Check sheet for the modelled part. Datum: model origin and axes. Units: mm. A direction names the side the tool comes from. Round coordinates to 2 decimals unless told otherwise and drop trailing zeros. Loops run counter-clockwise (first coordinate to the right, second up) from the corner with the lowest first, then second, coordinate; pieces in that order, holes last. Notation, with made-up numbers: (33.5, 43) - (92.5, 43) arc R24 ccw to (92.5, 69) - close; hole circle Ø8 at (24.5, -33.5). An arc over 180 degrees is marked (long way). Answer in a Markdown table with one row per item. Add a question column.
(1) Cross-section at C-C on y = 53. Enter the section's corners in (x, z) (3 decimals), then the cut area to 3 significant figures.
(2) Cross-section at A-A on z = 5. Enter the section's corners in (x, y) (3 decimals), then the cut area to 3 significant figures.
(3) Mould release check, pull along X, two halves, no side actions. Record for faces 5 (the flat face through (0, -63.5, 0)), 6 (the flat face through (-41.275, -1, 0)), 7 (the cylindrical face through (42.6, -0.4, 41.4)): +X half, -X half, draft (parallel to the pull), parting line (faces both ways), or undercut.
(4) Gauge pin test, flat ends, axial feed: pin 1 (4 mm diameter, centred on y = -5.5, z = 41.5, fed in from +X); pin 2 (2.5 mm diameter, centred on x = 85, y = -0.5, fed in from -Z); pin 3 (1.5 mm diameter, centred on y = 18.5, z = 41, fed in from -X). Record the tip position at first contact, or that the pin passes through.
(5) Access from +Z, -Z, +X, -X, +Y, -Y to the whole of each face (thin tool, end or side, straight path). Record for faces 1 (the flat face through (57, 0, 42.875)), 2 (the flat face through (80, 0, 38.1)), 3 (the flat face through (47, 25.4, 48)), 4 (the cylindrical face through (29.39, -16.79, 55.13)).
(6) Thickness scan on line 1 along Z through (x, y) = (34.5, -50) (3 decimals); line 2 along Y through (x, z) = (25, 45); line 3 along X through (y, z) = (9, 27.5) (3 decimals). Record the ranges inside material, lowest first.
(7) Cross-section at D-D on y = -10. Enter the section's corners in (x, z) (3 decimals), then the cut area to 3 significant figures.
(8) Cross-section at B-B on x = 65. Enter the section's corners in (y, z) (1 decimal), then the cut area to 3 significant figures.
from build123d import *

# Parameters (mm, degrees)
F1_DEPTH = 63.5
F2_DEPTH = 25.4
F3_DEPTH = 7.9375
F5_R     = 6.35


with BuildPart() as f1:
    # F0 (on Front) → F1 (new body, symmetric)
    with BuildSketch(Plane.XZ):
        Polygon((41.275, -9.525), (41.275, 9.525), (22.225, 9.525), (-41.275, 9.525), (-41.275, -9.525), align=None)
    extrude(amount=F1_DEPTH, both=True)

    # F0 (on Front) → F2 (join, symmetric)
    with BuildSketch(Plane.XZ):
        with BuildLine():
            Line((22.225, 9.525), (41.275, 9.525))
            Line((41.275, 9.525), (41.275, 38.1))
            ThreePointArc((41.275, 38.1), (42.673624, 41.476576), (46.0502, 42.8752))
            Line((46.0502, 42.8752), (60.325, 42.8752))
            Line((60.325, 42.8752), (60.325, 61.9252))
            Line((60.325, 61.9252), (46.0502, 61.9252))
            ThreePointArc((46.0502, 61.9252), (29.20324, 54.94696), (22.225, 38.1))
            Line((22.225, 38.1), (22.225, 9.525))
        make_face()
        Polygon((60.325, 61.9252), (60.325, 42.8752), (76.285926, 42.8752), (86.96812, 42.8752), (85.725, 61.9252), align=None)
    extrude(amount=F2_DEPTH, both=True)

    # F0 (on Front) → F3 (join, symmetric)
    with BuildSketch(Plane.XZ):
        with BuildLine():
            Line((-41.275, 9.525), (22.225, 9.525))
            Line((22.225, 9.525), (22.225, 38.1))
            ThreePointArc((22.225, 38.1), (29.20324, 54.94696), (46.0502, 61.9252))
            add(Edge.make_bspline(
                [(-41.275, 9.525), (-12.033702, 9.525), (10.122908, 69.295764), (46.0502, 61.9252)],
                knots=[0, 0, 0, 0, 101.840422, 101.840422, 101.840422, 101.840422], degree=3))
        make_face()
    extrude(amount=F3_DEPTH, both=True)

    # F0 (on Front) → F4 (revolve)
    with BuildSketch(Plane.XZ):
        Polygon((85.725, 66.675), (85.725, 61.9252), (86.96812, 42.8752), (86.96812, 38.1), (111.125, 38.1), (111.125, 66.675), align=None)
    revolve(axis=Axis((85.725, 0, 64.3001), (0, 0, 1)))

    # F5
    f5_edges = [f1.edges().sort_by_distance(p)[0] for p in [
        (-41.275, -63.5, 0),
        (41.275, -63.5, 0),
        (41.275, 63.5, 0),
        (-41.275, 63.5, 0),
    ]]
    fillet(f5_edges, radius=F5_R)


solid = f1.part
Answers:
| question | item | result |
|---|---|---|
| 1 | outline | (-41.275, -9.525) - (41.275, -9.525) - (41.275, 9.525) - (-41.275, 9.525) - close |
| 1 | area | 1,570 mm^2 |
| 2 | outline | (-41.275, -57.15) arc R6.35 ccw to (-34.925, -63.5) - (34.925, -63.5) arc R6.35 ccw to (41.275, -57.15) - (41.275, 57.15) arc R6.35 ccw to (34.925, 63.5) - (-34.925, 63.5) arc R6.35 ccw to (-41.275, 57.15) - close |
| 2 | area | 10,400 mm^2 |
| 3 | face 5 | draft |
| 3 | face 6 | -X half |
| 3 | face 7 | undercut |
| 4 | pin 1 | stops at x = 110.88 |
| 4 | pin 2 | stops at z = 38.1 |
| 4 | pin 3 | stops at x = 22.32 |
| 5 | face 1 | -Z |
| 5 | face 2 | -Z, +X, +Y, -Y |
| 5 | face 3 | +Z, +X, -X, +Y |
| 5 | face 4 | +Z, -X, -Y |
| 6 | line 1 | z = -9.525 to 9.525 |
| 6 | line 2 | y = -25.4 to 25.4 |
| 6 | line 3 | x = 22.225 to 41.275 |
| 7 | outline | (-41.275, -9.525) - (41.275, -9.525) - (41.275, 38.1) arc R4.775 cw to (46.05, 42.875) - (62.376, 42.875) - (62.376, 38.1) - (109.074, 38.1) - (109.074, 66.675) - (62.376, 66.675) - (62.376, 61.925) - (46.05, 61.925) arc R23.825 ccw to (22.225, 38.1) - (22.225, 9.525) - (-41.275, 9.525) - close |
| 7 | area | 4,190 mm^2 |
| 8 | outline | (-25.4, 42.9) - (-14.7, 42.9) - (-14.7, 38.1) - (14.7, 38.1) - (14.7, 42.9) - (25.4, 42.9) - (25.4, 61.9) - (14.7, 61.9) - (14.7, 66.7) - (-14.7, 66.7) - (-14.7, 61.9) - (-25.4, 61.9) - close |
| 8 | area | 1,250 mm^2 |
